Autodesk Inventor part; units mm, degrees
ref_plane "YZ Plane" through (0, 0, 0) normal (1, 0, 0) x (0, 1, 0)
ref_plane "XZ Plane" through (0, 0, 0) normal (0, 1, 0) x (-1, 0, 0)
ref_plane "XY Plane" through (0, 0, 0) normal (0, 0, 1) x (1, 0, 0)
sketch "Sketch1" plane through (0, 0, 0) normal (1, 0, 0) x (0, 1, 0)
  line L0 (-17.4625, 9.525) -> (17.4625, 9.525)
  line L1 (17.4625, 9.525) -> (17.4625, -9.525)
  line L2 (17.4625, -9.525) -> (-17.4625, -9.525)
  line L3 (-17.4625, -9.525) -> (-17.4625, 9.525)
  line L4 (-17.4625, 9.525) -> (17.4625, -9.525) construction
  line L5 (17.4625, 9.525) -> (-17.4625, -9.525) construction
  line L6 (3.175, -9.525) -> (3.175, 0)
  line L7 (3.175, 0) -> (-3.175, 0)
  line L8 (-3.175, 0) -> (-3.175, -9.525)
  line L9 (-17.4625, 9.525) -> (0, 9.525)
  line L10 (0, 9.525) -> (0, 98.425)
  line L11 (0, 98.425) -> (-17.4625, 98.425)
  line L12 (-17.4625, 98.425) -> (-17.4625, 9.525)
  line L13 (0, -9.525) -> (-0.0003, -140.97) construction
  line L14 (-0.0003, -140.97) -> (69.3079, -140.97)
  point P0 (0, 0)
  point P1 (0, 0)
  dimension "d0" = 6.35
  dimension "d1" = 9.525
  dimension "d2" = 9.525
  dimension "d3" = 19.05
  dimension "d4" = 34.925
  dimension "d5" = 0
  dimension "d6" = 88.9
  dimension "d7" = 131.445
revolve "Revolution1" add sketch "Sketch1" angle 60 mid plane about axis through (0, -0.0003, -140.97) along (0, 1, 0) contours L12 L11 L10 L0 | L0 L1 L2 L6 L7 L8 L3
sketch "Sketch2" plane through (-75.2475, 17.4625, -10.6375) normal (0, 1, 0) x (0.866, 0, 0.5)
  arc A0 (70.485, 28.4114) -> (122.0836, 80.01) centre (0, 150.495) ccw
  arc A1 (0, 19.05) -> (113.8347, 84.7725) centre (0, 150.495) ccw
  line L0 (0, 19.05) -> (0, 0) construction
  line L1 (113.8347, 84.7725) -> (122.0836, 80.01) construction
  arc A2 (89.2238, 47.5795) -> (117.9592, 82.3912) centre (0, 150.495) ccw construction
  circle A3 centre (11.8618, 14.805) radius 3.175
  circle A4 centre (68.0955, 32.5311) radius 3.175
  circle A5 centre (111.5692, 72.3618) radius 3.175
  point P0 (0, 0)
  dimension "d22" = 140.97
  dimension "d23" = 136.2075
  dimension "d24" = 6.35
  dimension "d25" = 11.8618
  dimension "d34" = 50
extrude "Extrusion2" cut sketch "Sketch2" against normal up to surface (14.2875 mm away)
sketch "Sketch3" plane through (0, 0, -140.97) normal (0, 1, 0) x (1, 0, 0)
  line L0 (-63.5, -212.9652) -> (63.5, -212.9652) construction
  line L1 (63.5, -212.9652) -> (63.5, -162.1652) construction
  line L2 (63.5, -162.1652) -> (-63.5, -162.1652) construction
  line L3 (-63.5, -162.1652) -> (-63.5, -212.9652) construction
  line L4 (-63.5, -212.9652) -> (63.5, -162.1652) construction
  line L5 (63.5, -212.9652) -> (-63.5, -162.1652) construction
  line L6 (-75.2475, -130.3325) -> (-119.6975, -207.3222)
  line L7 (75.2475, -130.3325) -> (119.6975, -207.3222)
  arc A0 (-97.4725, -168.8273) -> (97.4725, -168.8273) centre (0, 75.3248) ccw construction
  circle A1 centre (63.5, -162.1652) radius 3.175
  circle A2 centre (-63.5, -162.1652) radius 3.175
  circle A3 centre (63.5, -212.9652) radius 3.175
  circle A4 centre (-63.5, -212.9652) radius 3.175
  point P0 (0, -140.97)
  point P1 (0, -187.5652)
  dimension "d37" = 50.8
  dimension "d38" = 127
  dimension "d39" = 262.89
  dimension "d41" = 6.35
  dimension "d44" = 127
  dimension "d47" = 50.8
extrude "Extrusion3" cut sketch "Sketch3" against normal through all
equation "\"d2\" = d1"
equation "\"d3\" = 2 * d1"
properties part number "shelf_attachment" material "Aluminum 6061"
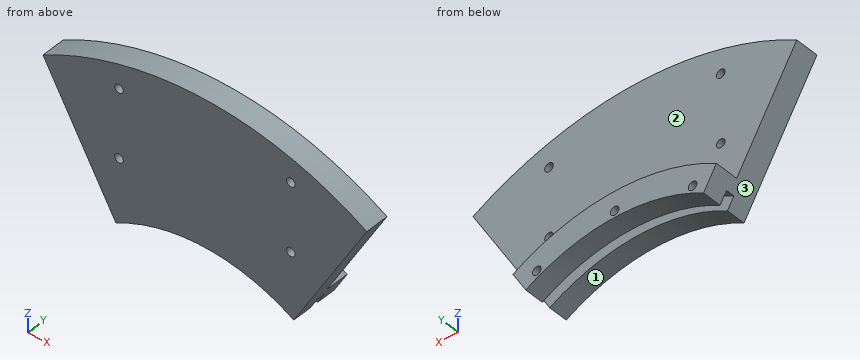
The model under review builds one solid part; all positions refer to its coordinate system, in mm. Face numbers are marked on the shaded views. Coordinates: 2 decimals unless noted, no trailing zeros. Loops run counter-clockwise (first coordinate to the right, second up) from the corner with the lowest first, then second, coordinate; pieces in that order, holes last. Notation, with made-up numbers: (42.25, -25) -> (50.25, -25) arc R17 ccw to (50.25, -5) -> close; hole circle Ø3 at (-29.75, 71.25). An arc over 180 degrees is marked (long way). Use a Markdown table: item, result. Add a question column.
1. Add section A-A on x = 63.5. Write out the cut boundary in (y, z) (1 decimal).
2. Draft analysis for pull direction X (two halves, no side actions). For the marked faces 1, 2 and 3, state which applies: pulls with the +X half, pulls with the -X half, needs draft (parallel to the pull), parting line crosses it, or undercut.
3. Add section B-B on y = 14.5. Give the number of separate pieces and of enclosed holes in the cut face, plus the area to 3 significant figures.
4. To check wall thickness, follow line 1 (Z direction, x = 63.5, y = -12.25); line 2 (X direction, y = -4, z = 20); line 3 (Y direction, x = 40.5, z = 76). State the ranges of each line that lie inside material, in increasing order.
5. Clearance check with flat-ended pins moving along their axes: pin 1 Ø5 at (x, y) = (-39, 11) entering from -Z; pin 2 Ø3 at (y, z) = (-9, 38) entering from +X; pin 3 Ø21.5 at (x, z) = (-3.5, -16.5) entering from -Y; pin 4 Ø5 at (x, z) = (63.5, 72) entering from +Y. State where each tip first meets the part, or that it passes through.
6. Add section D-D on x = 39.5. Write out the cut boundary in (y, z) (1 decimal).
Returned:
| question | item | result |
|---|---|---|
| 1 | outline | (-17.5, -25.9) -> (-3.2, -25.9) -> (-3.2, -15.1) -> (3.2, -15.1) -> (3.2, -25.9) -> (17.5, -25.9) -> (17.5, -4.5) -> (0, -4.5) -> (0, 18) -> (-17.5, 18) -> close; (-17.5, 24.4) -> (0, 24.4) -> (0, 68.8) -> (-17.5, 68.8) -> close; (-17.5, 75.2) -> (0, 75.2) -> (0, 89.8) -> (-17.5, 89.8) -> close |
| 2 | face 1 | undercut |
| 2 | face 2 | needs draft |
| 2 | face 3 | pulls with the -X half |
| 3 | separate pieces | 1 |
| 3 | enclosed holes | 3 |
| 3 | area | 2,720 mm² |
| 4 | line 1 | z = -25.88 to 18.02, 24.37 to 68.82, 75.17 to 89.85 |
| 4 | line 2 | x = -92.94 to -66.44, -60.56 to 60.56, 66.44 to 92.94 |
| 4 | line 3 | y = -17.46 to 0 |
| 5 | pin 1 | stops at z = -16.25 |
| 5 | pin 2 | stops at x = 104.19 |
| 5 | pin 3 | stops at y = -17.46 |
| 5 | pin 4 | passes through |
| 6 | outline | (-17.5, -15.6) -> (-3.2, -15.6) -> (-3.2, -5.6) -> (3.2, -5.6) -> (3.2, -15.6) -> (17.5, -15.6) -> (17.5, 4.2) -> (0, 4.2) -> (0, 95.1) -> (-17.5, 95.1) -> close |
